from build123d import *

# Parameters (mm, degrees)
BOSS_EXTRUDE1_DEPTH        = 10
M4_TAPPED_HOLE1_AT_2_COUNT = 2
M4_TAPPED_HOLE1_AT_2_PITCH = 113
SKETCH7_R                  = 4
CUT_EXTRUDE1_DEPTH         = 10
CUT_EXTRUDE1_DEPTH_BACK    = 6.6


with BuildPart() as part:
    # Sketch1 → Boss-Extrude1 (new body)
    with BuildSketch(Plane(origin=(0, 0, 0), x_dir=(0, 0, -1), z_dir=(1, 0, 0))):
        with BuildLine():
            Line((-61.001524227, 2), (-51.961524227, 2))
            ThreePointArc((-51.961524227, 2), (0, 52), (51.961524227, 2))
            Line((51.961524227, 2), (60.998475773, 2))
            Line((60.998475773, 2), (60.998475773, 17))
            Line((60.998475773, 17), (55.497747702, 17))
            ThreePointArc((55.497747702, 17), (54.620689683, 17.283131383), (54.07472853, 18.025641026))
            ThreePointArc((54.07472853, 18.025641026), (0, 57), (-54.07472853, 18.025641026))
            ThreePointArc((-54.07472853, 18.025641026), (-54.620689683, 17.283131383), (-55.497747702, 17))
            Line((-55.497747702, 17), (-61.001524227, 17))
            Line((-61.001524227, 17), (-61.001524227, 2))
        make_face()
    extrude(amount=BOSS_EXTRUDE1_DEPTH)

    # Sketch4 → M4 Tapped Hole1 (revolve, cut)
    with BuildSketch(Plane(origin=(5, 17, -56.498475773), x_dir=(0, 0, 1), z_dir=(1, 0, 0))):
        Polygon((0, 0), (0, 21.091420021), (1.65, 20.1), (1.65, 0), align=None)
    m4_tapped_hole1 = revolve(axis=Axis((5, 23.35, -56.498475773), (0, -1, 0)), mode=Mode.SUBTRACT)

    # M4 Tapped Hole1 at 2: M4 Tapped Hole1 ×2
    with Locations(*[(0, 0, i * M4_TAPPED_HOLE1_AT_2_PITCH) for i in range(1, M4_TAPPED_HOLE1_AT_2_COUNT)]):
        add(m4_tapped_hole1, mode=Mode.SUBTRACT)

    # Sketch7 → Cut-Extrude1 (cut, two sides)
    with BuildSketch(Plane(origin=(0, 17, 0), x_dir=(1, 0, 0), z_dir=(0, 1, 0))) as cut_extrude1_sk:
        with Locations((5, 56.498475773)):
            Circle(SKETCH7_R)
        with Locations((5, -56.501524227)):
            Circle(SKETCH7_R)
    extrude(amount=CUT_EXTRUDE1_DEPTH, mode=Mode.SUBTRACT)
    extrude(cut_extrude1_sk.sketch, amount=-CUT_EXTRUDE1_DEPTH_BACK, mode=Mode.SUBTRACT)


solid = part.part
Part model, mm, in its own coordinate system. A direction names the side the tool comes from. Give positions to 0.01 mm unless a question says otherwise; leave off trailing zeros. Loops run counter-clockwise (first coordinate to the right, second up) from the corner with the lowest first, then second, coordinate; pieces in that order, holes last.
(1) Drill centre lines: line 1 along Z through (x, y) = (5, 14.75); line 2 along Z through (x, y) = (5, 13.25); line 3 along Z through (x, y) = (5, 18.5). Where is each one in solid material? Low to high.
Return value:
line 1: z = -61 to -60.5, -52.5 to -49.86, 49.86 to 52.5, 60.5 to 61
line 2: z = -61 to -60.5, -52.5 to -50.28, 50.28 to 52.5, 60.5 to 61
line 3: z = -52.5 to -48.6, 48.6 to 52.5
(2) Band-saw the part on D-D (z = 0). Write the cut outline in (x, y), and give its area (3 significant figures).
Return value:
outline: (0, 52) - (10, 52) - (10, 57) - (0, 57) - close
area: 50.0 mm2
(3) Band-saw the part on A-A (x = 5). Write the cut outline in (y, z).
Return value:
outline: (2, -61) - (17, -61) - (17, -60.5) - (10.4, -60.5) - (10.4, -58.15) - (2, -58.15) - close; (2, -54.85) - (10.4, -54.85) - (10.4, -52.5) - (22.2, -52.5) arc R57 ccw to (22.19, 52.5) - (10.4, 52.5) - (10.4, 54.85) - (2, 54.85) - (2, 51.96) arc R52 cw to (2, -51.96) - close; (2, 58.15) - (10.4, 58.15) - (10.4, 60.5) - (17, 60.5) - (17, 61) - (2, 61) - close
(4) Pull direction Z, two halves, no side cores. Call faces 1 (the flat face through (5, 2, -54)), 2 (the flat face through (5, 10, 61.002)), 3 (the cylindrical face through (4.927, 6.259, -58.147)): pulls with the +Z half, pulls with the -Z half, needs draft (parallel to the pull), parting line crosses it, or undercut.
Return value:
face 1: needs draft
face 2: pulls with the +Z half
face 3: undercut
(5) Band-saw the part on B-B (y = 14). Write the cut outline in (x, z).
Return value:
outline: (0, -61) - (10, -61) - (10, -50.08) - (0, -50.08) - close; (0, 50.08) - (10, 50.08) - (10, 61) - (0, 61) - close; hole circle Ø8 at (5, -56.5); hole circle Ø8 at (5, 56.5)
(6) Pin check, flat tips, straight feed: pin 1 (2 mm diameter, centred on x = 5, z = 56.5, fed in from -Y); pin 2 (4 mm diameter, centred on x = 8.5, y = 40, fed in from -Z); pin 3 (4 mm diameter, centred on x = 5, z = -56.5, fed in from +Y); pin 4 (6 mm diameter, centred on x = 8, y = 32, fed in from +Z). Stop position of each tip, or through.
Return value:
pin 1: passes through
pin 2: stops at z = -42.49
pin 3: stops at y = 10.4
pin 4: stops at z = 49.07
(7) Band-saw the part on C-C (y = 44). Write the cut outline in (x, z), and give its area (3 significant figures).
Return value:
outline: (0, -36.24) - (10, -36.24) - (10, -27.71) - (0, -27.71) - close; (0, 27.71) - (10, 27.71) - (10, 36.24) - (0, 36.24) - close
area: 170 mm2
(8) 3-axis set-ups, long thin cutter, end or side, ignore diameter. For faces 4 (the cylindrical face through (4.927, 6.259, 54.853)), 5 (the flat face through (4.9, 17, -60.7)), 6 (the cylindrical face through (4.93, 56.99, -1)), 7 (the flat face through (4.9, 17, 60.7)), 8 (the flat face through (7, 10.4, -57)): which of +Z, -Z, +X, -X, +Y, -Y reach the whole face in a straight line?
Return value:
face 4: +Y, -Y
face 5: -Z, +X, -X, +Y
face 6: +X, -X, +Y
face 7: +Z, +X, -X, +Y
face 8: +Y
